Input: part model. Units: mm. Frame: model coordinates. A direction names the side the tool comes from. Round coordinates to 2 decimals unless told otherwise and drop trailing zeros. Loops run counter-clockwise (first coordinate to the right, second up) from the corner with the lowest first, then second, coordinate; pieces in that order, holes last.
1) Access query for faces 1 (the face through (25.26, 3, -47)), 2 (the face through (11.74, 3, 54)), 3 (the face through (-7.74, 3, -53)). Directions: +Z, -Z, +X, -X, +Y, -Y. A direction counts if a zero-diameter tool reaches every point of the face in a straight line with its end or side. Return the directions, or none.
2) Section B-B, the plane z = -59. Return loops of the section in (x, y), and give its area (3 significant figures).
3) Section A-A, the plane y = 5.5. Return loops of the section in (x, z).
4) Ray query, line 1 along Z through (x, y) = (-39.5, 3); line 2 along X through (y, z) = (3.75, -39). Return the intervals inside material, ascending.
5) Section C-C, the plane x = -35.5. Return loops of the section in (y, z), and give its area (3 significant figures).
6) First-contact query: pin 1 (2 mm diameter, centred on y = 5, z = -64.5, fed in from -X); pin 2 (2 mm diameter, centred on y = 3.5, z = 53, fed in from -X); pin 3 (2 mm diameter, centred on y = 3, z = 49.5, fed in from +X); pin 4 (1 mm diameter, centred on x = 17, z = 18, fed in from -Y). Flat tips, straight axial feed; report the tip coordinate or a pass-through.
from build123d import *

# Parameters (mm, degrees)
BOSS_EXTRUDE1_DEPTH = 7
SKETCH2_R           = 30
BOSS_EXTRUDE2_DEPTH = 7


with BuildPart() as part:
    # Sketch1 → Boss-Extrude1 (new body)
    with BuildSketch(Plane(origin=(0, 0, 0), x_dir=(1, 0, 0), z_dir=(0, 1, 0))):
        Polygon((-77.26, -11.74), (-77.26, 22.26), (-7.74, 22.26), (-7.74, 77.26), (25.26, 77.26), (25.26, 7.74), (81.26, 7.74), (81.26, -25.26), (11.74, -25.26), (11.74, -81.26), (-22.26, -81.26), (-22.26, -11.74), align=None)
        with BuildLine():
            Line((-1.65, 1.3), (1.65, 1.3))
            ThreePointArc((1.65, 1.3), (2.188477631, 0), (1.65, -1.3))
            Line((1.65, -1.3), (-1.65, -1.3))
            ThreePointArc((-1.65, -1.3), (-2.188477631, 0), (-1.65, 1.3))
        make_face(mode=Mode.SUBTRACT)
    extrude(amount=BOSS_EXTRUDE1_DEPTH)

    # Sketch2 → Boss-Extrude2 (add)
    with BuildSketch(Plane(origin=(0, 0, 0), x_dir=(1, 0, 0), z_dir=(0, 1, 0))):
        Circle(SKETCH2_R)
    extrude(amount=BOSS_EXTRUDE2_DEPTH)


solid = part.part
Final values:
1. face 1: -Z, +X, +Y, -Y
1. face 2: +Z, +X, +Y, -Y
1. face 3: -Z, -X, +Y, -Y
2. outline: (-7.74, 0) - (25.26, 0) - (25.26, 7) - (-7.74, 7) - close
2. area: 231 mm2
3. outline: (-77.26, -22.26) - (-20.11, -22.26) arc R30 ccw to (-7.74, -28.98) - (-7.74, -77.26) - (25.26, -77.26) - (25.26, -16.18) arc R30 ccw to (28.98, -7.74) - (81.26, -7.74) - (81.26, 25.26) - (16.18, 25.26) arc R30 ccw to (11.74, 27.61) - (11.74, 81.26) - (-22.26, 81.26) - (-22.26, 20.11) arc R30 ccw to (-27.61, 11.74) - (-77.26, 11.74) - close
4. line 1: z = -22.26 to 11.74
4. line 2: x = -7.74 to 25.26
5. outline: (0, -22.26) - (7, -22.26) - (7, 11.74) - (0, 11.74) - close
5. area: 238 mm2
6. pin 1: stops at x = -7.74
6. pin 2: stops at x = -22.26
6. pin 3: stops at x = 11.74
6. pin 4: stops at y = 0
